Part print with two shaded views. Sizes in mm from the minimum x, y, z corner. A direction names the side the tool comes from. Round coordinates to 2 decimals unless told otherwise and drop trailing zeros. Write each loop counter-clockwise with the first axis right and the second up, starting at its lowest first coordinate (ties: lowest second). Pieces come first, ordered by that corner, then holes.
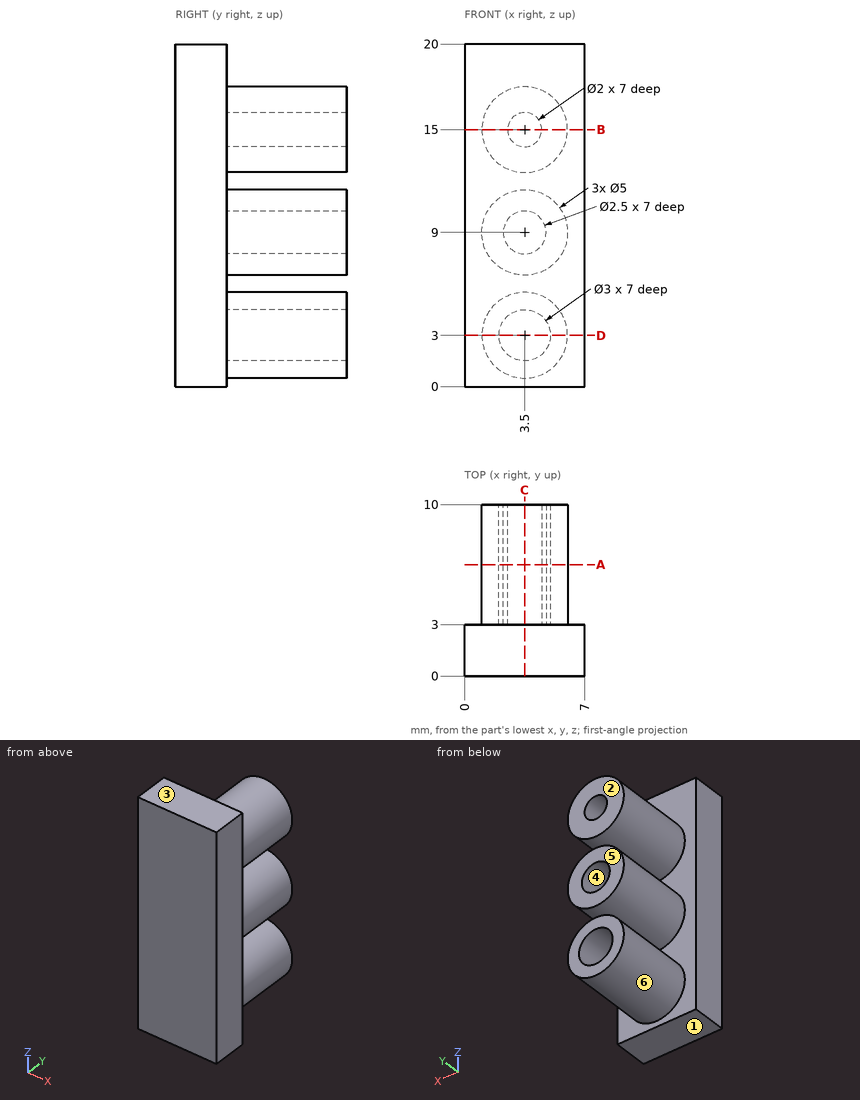
Q1. Mould opens along Z. For the marked faces 1, 2, 3 and 4 say: +Z half, -Z half, draft (parallel to the pull), parting line (faces both ways), or undercut.
Values follow:
face 1: -Z half
face 2: draft
face 3: +Z half
face 4: undercut
Q2. Cut at D-D on z = 3. Write the cut outline in (x, y), plus the area to 3 significant figures.
Values follow:
outline: (0, 0) - (7, 0) - (7, 3) - (6, 3) - (6, 10) - (5, 10) - (5, 3) - (2, 3) - (2, 10) - (1, 10) - (1, 3) - (0, 3) - close
area: 35.0 mm2
Q3. Cut at A-A on y = 6.5. Write the cut outline in (x, z).
Values follow:
outline: circle Ø5 at (3.5, 3); circle Ø5 at (3.5, 9); circle Ø5 at (3.5, 15); hole circle Ø3 at (3.5, 3); hole circle Ø2.5 at (3.5, 9); hole circle Ø2 at (3.5, 15)
Q4. Drop flat-ended pins along their axis: pin 1 (2 mm diameter, centred on x = 6, y = 7, fed in from -Z); pin 2 (2 mm diameter, centred on y = 7, z = 4, fed in from -X); pin 3 (1.5 mm diameter, centred on x = 4, z = 2.5, fed in from +Y). Give the stop position or say it passes through.
Values follow:
pin 1: stops at z = 1
pin 2: stops at x = 1
pin 3: stops at y = 3
Q5. Which spindle directions (+Z, -Z, +X, -X, +Y, -Y) get a long thin tool onto all of the face, cutting with end or side? Do the marked faces 5 and 6. Say none if no direction does.
Values follow:
face 5: +Z, -Z, +X, -X, +Y
face 6: +Y
Q6. Cut at C-C on x = 3.5. Write the cut outline in (y, z), plus the area to 4 significant figures.
Values follow:
outline: (0, 0) - (3, 0) - (3, 0.5) - (10, 0.5) - (10, 1.5) - (3, 1.5) - (3, 4.5) - (10, 4.5) - (10, 5.5) - (3, 5.5) - (3, 6.5) - (10, 6.5) - (10, 7.75) - (3, 7.75) - (3, 10.25) - (10, 10.25) - (10, 11.5) - (3, 11.5) - (3, 12.5) - (10, 12.5) - (10, 14) - (3, 14) - (3, 16) - (10, 16) - (10, 17.5) - (3, 17.5) - (3, 20) - (0, 20) - close
area: 112.5 mm2
Q7. Wall check: L1, parallel to Z at x = 3.5, y = 4.5; L2, parallel to X at y = 8.75, z = 3; L3, parallel to X at y = 5.5, z = 15. Give the ranges that are in metal, low to high.
Values follow:
L1: z = 0.5 to 1.5, 4.5 to 5.5, 6.5 to 7.75, 10.25 to 11.5, 12.5 to 14, 16 to 17.5
L2: x = 1 to 2, 5 to 6
L3: x = 1 to 2.5, 4.5 to 6
Q8. Cut at B-B on z = 15. Write the cut outline in (x, y).
Values follow:
outline: (0, 0) - (7, 0) - (7, 3) - (6, 3) - (6, 10) - (4.5, 10) - (4.5, 3) - (2.5, 3) - (2.5, 10) - (1, 10) - (1, 3) - (0, 3) - close
